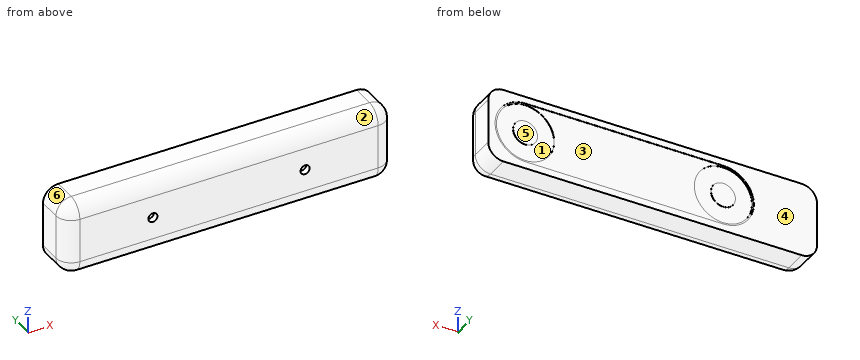
Autodesk Inventor part; units mm, degrees
ref_plane "YZ Plane" through (0, 0, 0) normal (1, 0, 0) x (0, 1, 0)
ref_plane "XZ Plane" through (0, 0, 0) normal (0, 1, 0) x (-1, 0, 0)
ref_plane "XY Plane" through (0, 0, 0) normal (0, 0, 1) x (1, 0, 0)
sketch "Sketch1" plane through (0, 0, 0) normal (0, 1, 0) x (-1, 0, 0)
  line L0 (0, 0) -> (0, -12.25)
  line L1 (0, -12.25) -> (54, -12.25)
  line L2 (54, -12.25) -> (54, 12.25)
  line L3 (54, 12.25) -> (-54, 12.25)
  line L4 (-54, 12.25) -> (-54, -12.25)
  line L5 (-54, -12.25) -> (0, -12.25)
  dimension "d0" = 12.25
  dimension "d1" = 54
  dimension "d2" = 24.5
  dimension "d3" = 108
  dimension "d4" = 24.5
extrude "Extrusion1" add sketch "Sketch1" along normal blind 12.5
fillet "Fillet1" radius 5 4 edges at (-54, 6.25, 12.25) (-54, 6.25, -12.25) (54, 6.25, 12.25) (54, 6.25, -12.25)
sketch "Sketch2" plane through (0, 12.5, 0) normal (0, 1, 0) x (1, 0, 0)
  line L0 (54, -7.25) -> (54, 7.25)
  line L1 (54, 0) -> (41.75, 0)
  circle A0 centre (41.75, 0) radius 10
  line L2 (41.75, 0) -> (-23.25, 0)
  circle A1 centre (-23.25, 0) radius 10
  line L3 (-23.25, 10) -> (41.75, 10)
  line L4 (-23.25, -10) -> (41.75, -10)
  point P0 (0, 0)
  dimension "d8" = 12.25
  dimension "d9" = 20
  dimension "d10" = 65
  dimension "d11" = 20
extrude "Extrusion2" cut sketch "Sketch2" against normal blind 0.1
sketch "Sketch3" plane through (0, 12.4, 0) normal (0, 1, 0) x (1, 0, 0)
  line L0 (-23.25, 10) -> (41.75, 10)
  arc A0 (-23.25, 10) -> (-23.25, -10) centre (-23.25, 0) ccw
  line L1 (41.75, -10) -> (-23.25, -10)
  arc A1 (41.75, -10) -> (41.75, 10) centre (41.75, 0) ccw
  circle A2 centre (-23.25, 0) radius 9.5
  circle A3 centre (41.75, 0) radius 9.5
  point P0 (0, 0)
  dimension "d14" = 19
  dimension "d15" = 19
extrude "Extrusion3" cut sketch "Sketch3" against normal blind 0.1 contours A2 | A3
sketch "Sketch4" plane through (-23.25, 12.3, 0) normal (0, 1, 0) x (1, 0, 0)
  circle A0 centre (0, 0) radius 9.5
  circle A1 centre (65, 0) radius 9.5
  circle A2 centre (0, 0) radius 4
  circle A3 centre (65, 0) radius 4
  point P0 (23.25, 0)
  dimension "d18" = 8
  dimension "d19" = 8
extrude "Extrusion4" add sketch "Sketch4" along normal blind 0.1 contours A2 | A3
fillet "Fillet2" radius 5 8 edges at (-52.5355, 0, -10.7855) (-54, 0, 0) (-52.5355, 0, 10.7855) (0, 0, 12.25) (52.5355, 0, 10.7855) (54, 0, 0) (52.5355, 0, -10.7855) (0, 0, -12.25)
sketch "Sketch5" plane through (0, 0, 0) normal (0, -1, 0) x (1, 0, 0)
  line L0 (0, 0) -> (-25, 0)
  line L1 (0, 0) -> (25, 0)
  circle A0 centre (25, 0) radius 1.5
  circle A1 centre (-25, 0) radius 1.5
  dimension "d23" = 25
  dimension "d24" = 25
  dimension "d25" = 3
  dimension "d26" = 3
extrude "Extrusion5" cut sketch "Sketch5" against normal blind 2
properties part number "IntelRealSenseT265"
Verification items for the finished model (mm, model axes). Face numbers are marked on the shaded views. A direction names the side the tool comes from. Give positions to 0.01 mm unless a question says otherwise; leave off trailing zeros. Order: outer loops, then holes, each group sorted by start corner. A loop starts at its lowest first (then second) coordinate and runs counter-clockwise, first axis right, second up. Notation, with made-up numbers: M 24,-15 L 55,-15 A24 ccw 55,5 Z; hole C 1.5,47 d1. An arc over 180 degrees is marked long. Use one line per item in the form item = value. Start each with the question number.
Q1. Section check A-A (x = 14.5). Enter the section's corners in (y, z), then the cut area to 3 significant figures.
Q2. Access from +Z, -Z, +X, -X, +Y, -Y to the whole of each face (thin tool, end or side, straight path). Record for the marked faces 1 and 2.
Q3. Section check C-C (x = 36). Enter the section's corners in (y, z), then the cut area to 3 significant figures.
Q4. Go/stop test with flat-tipped pins: pin 1 Ø11.5 at (x, z) = (-23.25, 0) entering from +Y; pin 2 Ø1.5 at (x, z) = (-24.5, -0.5) entering from -Y. Record where each tip stops, or that it passes through.
Q5. Scan lines: line 1 along Z through (x, y) = (41.75, 12.35); line 2 along Z through (x, y) = (-23.25, 12.45); line 3 along Z through (x, y) = (25, 0.6). Record each from-to range of solid material in increasing order. Write a range as [from, to].
Q6. Mould release check, pull along Z, two halves, no side actions. Record for the marked faces 3, 4, 5 and 6: +Z half, -Z half, draft (parallel to the pull), parting line (faces both ways), or undercut.
Q7. Section check D-D (x = -25). Enter the section's corners in (y, z), then the cut area to 3 significant figures.
Evaluation:
q1.outline = M 0,-7.25 A5 ccw 5,-12.25 L 12.5,-12.25 L 12.5,-10 L 12.4,-10 L 12.4,10 L 12.5,10 L 12.5,12.25 L 5,12.25 A5 ccw 0,7.25 Z
q1.area = 294 mm2
q2.face_1 = +Y
q2.face_2 = +Z, +X, -X, -Y
q3.outline = M 0,-7.25 A5 ccw 5,-12.25 L 12.5,-12.25 L 12.5,-10 L 12.4,-10 L 12.4,-7.56 L 12.3,-7.56 L 12.3,7.56 L 12.4,7.56 L 12.4,10 L 12.5,10 L 12.5,12.25 L 5,12.25 A5 ccw 0,7.25 Z
q3.area = 292 mm2
q4.pin_1 = 12.4
q4.pin_2 = 2
q5.line_1 = [-12.25, -9.5], [-4, 4], [9.5, 12.25]
q5.line_2 = [-12.25, -10], [10, 12.25]
q5.line_3 = [-9.62, -1.5], [1.5, 9.62]
q6.face_3 = undercut
q6.face_4 = draft
q6.face_5 = undercut
q6.face_6 = +Z half
q7.outline = M 0,-7.25 A5 ccw 5,-12.25 L 12.5,-12.25 L 12.5,-9.85 L 12.4,-9.85 L 12.4,-9.34 L 12.3,-9.34 L 12.3,-3.6 L 12.4,-3.6 L 12.4,3.6 L 12.3,3.6 L 12.3,9.34 L 12.4,9.34 L 12.4,9.85 L 12.5,9.85 L 12.5,12.25 L 5,12.25 A5 ccw 0,7.25 L 0,1.5 L 2,1.5 L 2,-1.5 L 0,-1.5 Z
q7.area = 286 mm2
